The listing builds one solid part. Answer for the finished solid, in the listing's coordinates (mm). A direction names the side the tool comes from. Give positions to 0.01 mm unless a question says otherwise; leave off trailing zeros. Write each loop counter-clockwise with the first axis right and the second up, starting at its lowest first coordinate (ties: lowest second). Pieces come first, ordered by that corner, then holes. Notation, with made-up numbers: (85.25, -35) -> (91.25, -35) arc R13 cw to (91.25, -26) -> close; hole circle Ø4 at (54, 63.25). An arc over 180 degrees is marked (long way). One line per question, with ' | ' between items.
from build123d import *

# Parameters (mm, degrees)
CUT_EXTRUDE1_REACH      = 173.895
CUT_EXTRUDE1_END_RADIUS = 7.5
SKETCH2_W               = 8
SKETCH2_H               = 13


with BuildPart() as part:
    # Sketch1 → Revolve1 (revolve)
    with BuildSketch(Plane.XY, mode=Mode.PRIVATE) as revolve1_sk:
        Polygon((127, 6.5), (127, 7.5), (55, 7.5), (55, 18), (-55, 18), (-55, 7.5), (-170, 7.5), (-170, 6.5), align=None)
    revolve(revolve1_sk.sketch.rotate(Axis((196.356223274, 0, 0), (-1, 0, 0)), 90), axis=Axis((196.356223274, 0, 0), (-1, 0, 0)))

    # Cut-Extrude1: up to this cylinder (the profile starts inside it)
    cut_extrude1_end = Plane(origin=(-64, 0, 0), z_dir=(1, 0, 0)) * Cylinder(CUT_EXTRUDE1_END_RADIUS, 363.79, mode=Mode.PRIVATE)
    # Sketch2 → Cut-Extrude1 (cut, up to the surface)
    with BuildSketch(Plane(origin=(0, 0, 0), x_dir=(1, 0, 0), z_dir=(0, 1, 0)), mode=Mode.PRIVATE) as cut_extrude1_sk1:
        with Locations((-64, 0)):
            Rectangle(SKETCH2_W, SKETCH2_H)
    cut_extrude1_tool1 = extrude(cut_extrude1_sk1.sketch, amount=-CUT_EXTRUDE1_REACH, mode=Mode.PRIVATE) & cut_extrude1_end
    add(cut_extrude1_tool1.solids().sort_by_distance((-64, 0, 0))[0], mode=Mode.SUBTRACT)


solid = part.part
Item 1: Flat-ended cylindrical pins translate along their axes: pin 1 (3 mm diameter, centred on x = -63, y = -2, fed in from -Z); pin 2 (12 mm diameter, centred on x = 37, z = 0, fed in from -Y); pin 3 (4 mm diameter, centred on y = -2.5, z = 3, fed in from -X); pin 4 (2 mm diameter, centred on x = -63.5, y = -4, fed in from -Z). Find the tip coordinate at first contact, or state that the pin passes through.
Answers below:
pin 1: z = -7.48 | pin 2: y = -18 | pin 3: through | pin 4: z = -6.87
Item 2: Find section B-B (x = -62.5). Write down the section's boundary in (y, z).
Answers below:
outline: (-3.74, -6.5) arc R7.5 ccw (long way) to (-3.74, 6.5) -> (0, 6.5) arc R6.5 cw to (0, -6.5) -> close
Item 3: Consider line 1 (Y direction, x = -43.5, z = 0); line 2 (Y direction, x = 64, z = 0); line 3 (Z direction, x = -58, y = -0.5). Determine where each line is inside the solid, lowest interval first. Write a range as [from, to].
Answers below:
line 1: [-18, -6.5], [6.5, 18] | line 2: [-7.5, -6.5], [6.5, 7.5] | line 3: [-7.48, -6.48], [6.48, 7.48]
Item 4: Find section A-A (z = 0). Write down the section's boundary in (x, y), then the cut area to 3 significant figures.
Answers below:
outline: (-170, -7.5) -> (-68, -7.5) -> (-68, -6.5) -> (-170, -6.5) -> close; (-170, 6.5) -> (127, 6.5) -> (127, 7.5) -> (55, 7.5) -> (55, 18) -> (-55, 18) -> (-55, 7.5) -> (-170, 7.5) -> close; (-60, -7.5) -> (-55, -7.5) -> (-55, -18) -> (55, -18) -> (55, -7.5) -> (127, -7.5) -> (127, -6.5) -> (-60, -6.5) -> close | area: 2,900 mm²
Item 5: Find section D-D (y = -10). Write down the section's boundary in (x, z), then the cut area to 3 significant figures.
Answers below:
outline: (-55, -14.97) -> (55, -14.97) -> (55, 14.97) -> (-55, 14.97) -> close | area: 3,290 mm²
Item 6: A tool of negligible diameter and unlimited length cuts with its end or side. For faces 1 (the face through (-55, 8, 0)), 2 (the face through (-68, -7, 0)), 3 (the face through (90.496, -6.324, -4.032)), from which of +Z, -Z, +X, -X, +Y, -Y can it reach the whole face along a straight path? Write none if from no direction.
Answers below:
face 1: -X | face 2: -Y | face 3: +X
Item 7: Determine the mould class of faces 4 (the face through (-170, -3, 6)), 5 (the face through (-60, -7, 0)), 6 (the face through (-113.3, 7.32, 1.63)) for opening direction Z: pulls with the +Z half, pulls with the -Z half, needs draft (parallel to the pull), parting line crosses it, or undercut.
Answers below:
face 4: needs draft | face 5: undercut | face 6: parting line crosses it
Item 8: Find section C-C (x = -139). Write down the section's boundary in (y, z), then the cut area to 3 significant figures.
Answers below:
outline: circle Ø15 at (0, 0); hole circle Ø13 at (0, 0) | area: 44.0 mm²
